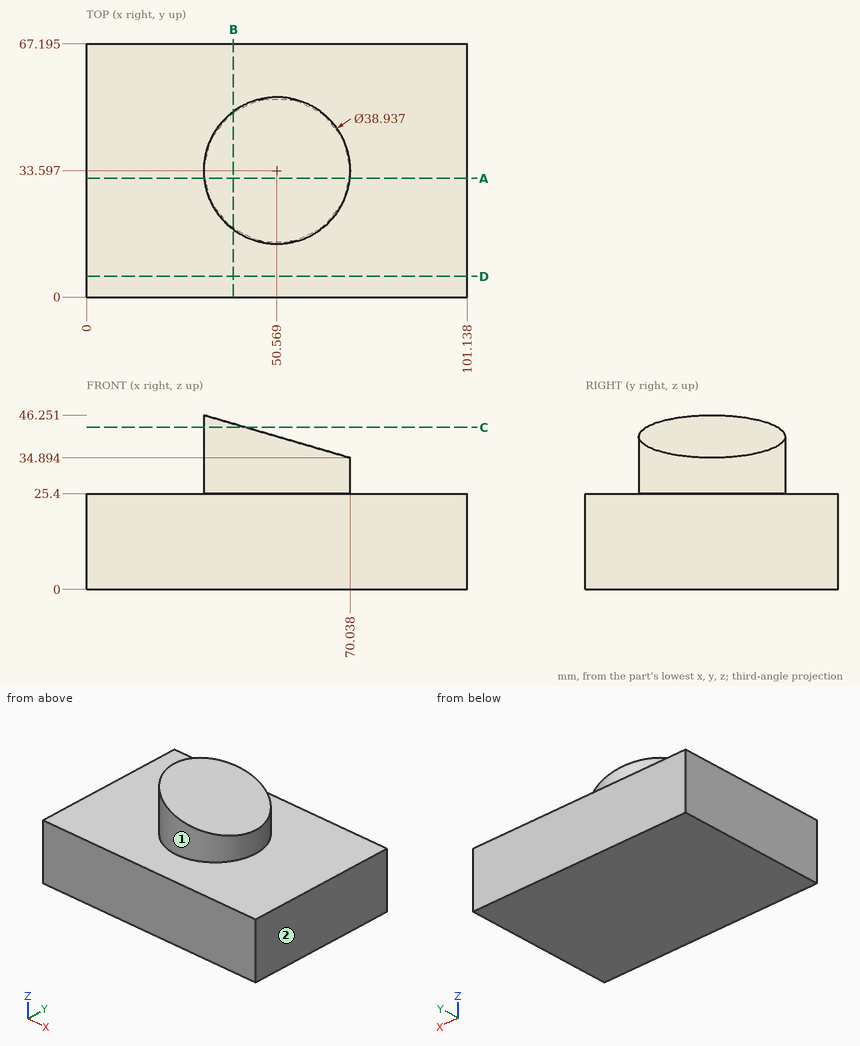
Job drawing, mm, ordinate dimensions from the low corner. One solid piece. A direction names the side the tool comes from. Coordinates: 2 decimals unless noted, no trailing zeros. Order: outer loops, then holes, each group sorted by start corner. A loop starts at its lowest first (then second) coordinate and runs counter-clockwise, first axis right, second up. Notation, with made-up numbers: (38.25, 75) - (71.25, 75) arc R11 ccw to (71.25, 82) - close; hole circle Ø9 at (46, 26). An arc over 180 degrees is marked (long way). Return JSON: item names as keys, results as strings. Group by question number.
1) Probe line 1 (Z direction, x = 70, y = 26.5); line 2 (Y direction, x = 36, z = 32) (1 decimal); line 3 (Z direction, x = 48.5, y = 43) (1 decimal). List the from-to ranges inside material, lowest first. Write a range as from..to.
2) Saw through at B-B, the plane x = 39. Write the cut outline in (y, z) (1 decimal).
3) Tool access for the marked faces 1 and 2: list every direction of +Z, -Z, +X, -X, +Y, -Y with a clear straight run to the whole face (end or side of a thin tool).
4) Saw through at D-D, the plane y = 5.5. Write the cut outline in (x, z), plus the area to 3 significant figures.
5) Saw through at C-C, the plane z = 43. Write the cut outline in (x, y).
6) Flat gauge pins, fed straight in: P1, Ø20, axis at x = 73, y = 42.5, coming from the +Z side; P2, Ø6, axis at y = 38, z = 29, coming from the +X side; P3, Ø12, axis at x = 37.5, y = 30, coming from the +Z side (1 decimal). Where does each tip first touch, or does it go through?
7) Saw through at A-A, the plane y = 31.5. Write the cut outline in (x, z) (1 decimal), plus the area to 3 significant figures.
Values found:
{
 "1": {"line 1": "z = 0..25.4", "line 2": "y = 20.7..46.5", "line 3": "z = 0..41.2"},
 "2": {"outline": "(0, 0) - (67.2, 0) - (67.2, 25.4) - (49.3, 25.4) - (49.3, 43.9) - (17.9, 43.9) - (17.9, 25.4) - (0, 25.4) - close"},
 "3": {"face 1": "+Z", "face 2": "+Z, -Z, +X, +Y, -Y"},
 "4": {"outline": "(0, 0) - (101.14, 0) - (101.14, 25.4) - (0, 25.4) - close", "area": "2,570 mm²"},
 "5": {"outline": "(42.25, 16) - (42.25, 51.2) arc R19.47 ccw to start"},
 "6": {"P1": "stops at z = 36.95", "P2": "stops at x = 69.99", "P3": "stops at z = 46.1"},
 "7": {"outline": "(0, 0) - (101.1, 0) - (101.1, 25.4) - (69.9, 25.4) - (69.9, 34.9) - (31.2, 46.2) - (31.2, 25.4) - (0, 25.4) - close", "area": "3,160 mm²"}
}
